Can you work these out from the model? Positions are in its coordinate system, mm. Give positions to 0.01 mm unless a question says otherwise; leave off trailing zeros. Loops run counter-clockwise (first coordinate to the right, second up) from the corner with the lowest first, then second, coordinate; pieces in that order, holes last. Notation, with made-up numbers: M 72.5,47.25 L 112.5,47.25 A29 ccw 112.5,75.25 Z; hole C 43.5,35 d10. An arc over 180 degrees is marked long. Put each result on its own line as item: value. Start each with the question number.
1) Imagine slicing it at D-D (x = -20). Write out the boundary of the cut face in (y, z).
2) For P1, Ø14, axis at x = -100, z = -100, coming from the +Y side; P2, Ø9, axis at x = -180, z = -50, coming from the -Y side, each with a flat end and sliding along its axis, tell me the tip position at first contact or that it passes through.
3) Please list where these lines run through material, in increasing order: line 1 along X through (y, z) = (4.25, -50); line 2 along Z through (x, y) = (-180, 3.45); line 3 along Z through (x, y) = (-17, 2.15). Write a range as from..to.
4) Imagine slicing it at B-B (z = -150). Write out the boundary of the cut face in (x, y), then the cut area to 3 significant figures.
5) Imagine slicing it at A-A (x = -100). Write out the boundary of the cut face in (y, z), then the cut area to 4 significant figures.
6) Imagine slicing it at C-C (y = 1.25). Write out the boundary of the cut face in (x, z), then the cut area to 3 significant figures.
from build123d import *

# Parameters (mm, degrees)
SKETCH1_W                                           = 200
SKETCH1_H                                           = 200
BOSS_EXTRUDE1_DEPTH                                 = 5
CSK_FOR_M5_COUNTERSUNK_FLAT_HEAD_SCREW1_D           = 5.5
CSK_FOR_M5_COUNTERSUNK_FLAT_HEAD_SCREW1_DEPTH       = 10
CSK_FOR_M5_COUNTERSUNK_FLAT_HEAD_SCREW1_CSINK_D     = 11.2
CSK_FOR_M5_COUNTERSUNK_FLAT_HEAD_SCREW1_CSINK_ANGLE = 90
CSK_FOR_M5_COUNTERSUNK_FLAT_HEAD_SCREW1_TIP         = 1.652366702
SKETCH5_R                                           = 11.75
CUT_EXTRUDE1_DEPTH                                  = 10


with BuildPart() as part:
    # Sketch1 → Boss-Extrude1 (new body)
    with BuildSketch(Plane(origin=(0, 0, 0), x_dir=(1, 0, 0), z_dir=(0, 1, 0))):
        with Locations((-100, 100)):
            Rectangle(SKETCH1_W, SKETCH1_H)
    extrude(amount=BOSS_EXTRUDE1_DEPTH)

    # CSK for M5 Countersunk Flat Head Screw1
    with Locations(Plane(origin=(0, 0, 0), x_dir=(-1, 0, 0), z_dir=(0, -1, 0))):
        with Locations((180, 50), (180, 150), (20, 50), (20, 150)):
            CounterSinkHole(CSK_FOR_M5_COUNTERSUNK_FLAT_HEAD_SCREW1_D / 2, CSK_FOR_M5_COUNTERSUNK_FLAT_HEAD_SCREW1_CSINK_D / 2, depth=CSK_FOR_M5_COUNTERSUNK_FLAT_HEAD_SCREW1_DEPTH, counter_sink_angle=CSK_FOR_M5_COUNTERSUNK_FLAT_HEAD_SCREW1_CSINK_ANGLE)
            with Locations((0, 0, -(CSK_FOR_M5_COUNTERSUNK_FLAT_HEAD_SCREW1_DEPTH + CSK_FOR_M5_COUNTERSUNK_FLAT_HEAD_SCREW1_TIP / 2))):  # 118° drill point
                Cone(0, CSK_FOR_M5_COUNTERSUNK_FLAT_HEAD_SCREW1_D / 2, CSK_FOR_M5_COUNTERSUNK_FLAT_HEAD_SCREW1_TIP, mode=Mode.SUBTRACT)

    # Sketch5 → Cut-Extrude1 (cut)
    with BuildSketch(Plane.XZ):
        with Locations((-100, -100)):
            Circle(SKETCH5_R)
    extrude(amount=-CUT_EXTRUDE1_DEPTH, mode=Mode.SUBTRACT)


solid = part.part
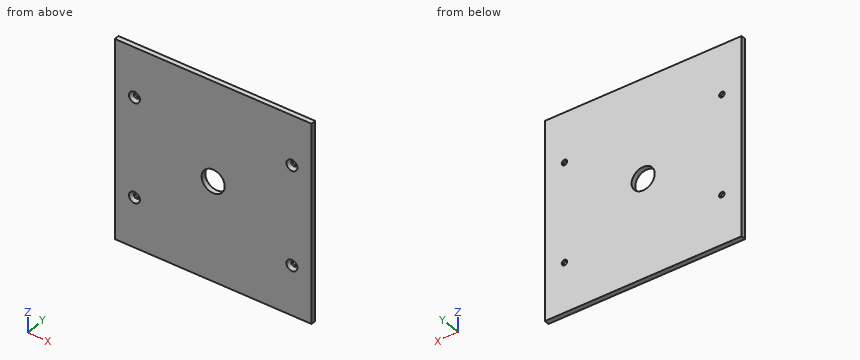
Recorded:
1. outline: M 0,-200 L 5,-200 L 5,-152.75 L 2.85,-152.75 L 0,-155.6 Z; M 0,-144.4 L 2.85,-147.25 L 5,-147.25 L 5,-52.75 L 2.85,-52.75 L 0,-55.6 Z; M 0,-44.4 L 2.85,-47.25 L 5,-47.25 L 5,0 L 0,0 Z
2. P1: through
2. P2: y = 1.1
3. line 1: -200..-182.75, -177.25..-22.75, -17.25..0
3. line 2: -200..-152.75, -147.25..-52.75, -47.25..0
3. line 3: -200..-151.7, -148.3..-51.7, -48.3..0
4. outline: M -200,0 L -185.6,0 L -182.75,2.85 L -182.75,5 L -200,5 Z; M -177.25,2.85 L -174.4,0 L -25.6,0 L -22.75,2.85 L -22.75,5 L -177.25,5 Z; M -17.25,2.85 L -14.4,0 L 0,0 L 0,5 L -17.25,5 Z
4. area: 929 mm²
5. outline: M 0,-200 L 5,-200 L 5,-111.75 L 0,-111.75 Z; M 0,-88.25 L 5,-88.25 L 5,0 L 0,0 Z
5. area: 882.5 mm²
6. outline: M -200,-200 L 0,-200 L 0,0 L -200,0 Z; hole C -180,-150 d8.7; hole C -180,-50 d8.7; hole C -100,-100 d23.5; hole C -20,-150 d8.7; hole C -20,-50 d8.7
6. area: 39,300 mm²
